Geometry: final body of the model. Coordinates: model frame, mm. A direction names the side the tool comes from. Coordinates: 2 decimals unless noted, no trailing zeros. Write each loop counter-clockwise with the first axis right and the second up, starting at its lowest first coordinate (ties: lowest second). Pieces come first, ordered by that corner, then holes. Notation, with made-up numbers: (-23, 80) -> (20, 80) arc R9 ccw to (20, 95) -> close; hole circle Ø4 at (31, 45). An arc over 180 degrees is marked (long way). One line per item, written item: value. Start each with the question number.
from build123d import *

# Parameters (mm, degrees)
SKETCH1_R             = 10.5
SKETCH1_R_2           = 7
BOSS_EXTRUDE1_DEPTH   = 90
SKETCH2_R             = 11.5
CUT_EXTRUDE1_DEPTH    = 6
SKETCH3_R             = 1.5
CUT_EXTRUDE2_DEPTH    = 40
SKETCH4_W             = 43
SKETCH4_H             = 44
CUT_EXTRUDE3_DEPTH    = 3
SKETCH5_R             = 11.5
CUT_EXTRUDE4_DEPTH    = 9
CIRPATTERN1_COUNT     = 4
SKETCH9_R             = 4
SKETCH9_R_2           = 5
CUT_EXTRUDE5_DEPTH    = 177.068168617
SKETCH10_R            = 12
CUT_EXTRUDE6_DEPTH    = 8
M4_TAPPED_HOLE1_D     = 3.3
M4_TAPPED_HOLE1_DEPTH = 19.008579979
M4_TAPPED_HOLE1_TIP   = 0.991420021


with BuildPart() as part:
    # Sketch1 → Boss-Extrude1 (new body)
    with BuildSketch(Plane.XY):
        with BuildLine():
            Line((0, 0), (64, 0))
            ThreePointArc((64, 0), (71.071067812, 2.928932188), (74, 10))
            Line((74, 10), (74, 122))
            ThreePointArc((74, 122), (71.071067812, 129.071067812), (64, 132))
            Line((64, 132), (0, 132))
            Line((0, 132), (0, 120))
            Line((0, 120), (40, 120))
            Line((40, 120), (40, 12))
            Line((40, 12), (0, 12))
            Line((0, 12), (0, 0))
        make_face()
        with Locations(Location((57, 106, 0), (0, 0, 180))):
            Circle(SKETCH1_R, mode=Mode.SUBTRACT)
        with Locations(Location((57, 66, 0), (0, 0, 180))):
            Circle(SKETCH1_R_2, mode=Mode.SUBTRACT)
        with Locations(Location((57, 26, 0), (0, 0, 180))):
            Circle(SKETCH1_R, mode=Mode.SUBTRACT)
    extrude(amount=BOSS_EXTRUDE1_DEPTH)

    # Sketch2 → Cut-Extrude1 (cut)
    with BuildSketch(Plane(origin=(0, 0, 0), x_dir=(-1, 0, 0), z_dir=(0, 0, -1))):
        with Locations((-57, 66)):
            Circle(SKETCH2_R)
    extrude(amount=-CUT_EXTRUDE1_DEPTH, mode=Mode.SUBTRACT)

    # Sketch3 → Cut-Extrude2 (cut)
    with BuildSketch(Plane(origin=(0, 0, 6), x_dir=(-1, 0, 0), z_dir=(0, 0, -1))):
        with Locations((-57, 74)):
            Circle(SKETCH3_R)
        with Locations((-49, 66)):
            Circle(SKETCH3_R)
        with Locations((-57, 58)):
            Circle(SKETCH3_R)
        with Locations((-65, 66)):
            Circle(SKETCH3_R)
    extrude(amount=-CUT_EXTRUDE2_DEPTH, mode=Mode.SUBTRACT)

    # Sketch4 → Cut-Extrude3 (cut)
    with BuildSketch(Plane(origin=(0, 132, 0), x_dir=(1, 0, 0), z_dir=(0, 1, 0))):
        with Locations((21.5, -45)):
            Rectangle(SKETCH4_W, SKETCH4_H)
    extrude(amount=-CUT_EXTRUDE3_DEPTH, mode=Mode.SUBTRACT)

    # Sketch5 → Cut-Extrude4 (cut)
    with BuildSketch(Plane(origin=(0, 129, 0), x_dir=(1, 0, 0), z_dir=(0, 1, 0))):
        with Locations(Location((21.5, -45, 0), (0, 0, 270))):
            Circle(SKETCH5_R)
    extrude(amount=-CUT_EXTRUDE4_DEPTH, mode=Mode.SUBTRACT)

    # Sketch7 → CBORE for M3 Pan Head Screw1 (revolve, cut)
    with BuildSketch(Plane(origin=(6, 120, 29.5), x_dir=(0, 0, -1), z_dir=(1, 0, 0))):
        Polygon((0, 0), (0, 21.021463052), (1.7, 20), (1.7, 3), (2.75, 3), (2.75, 0), align=None)
    cbore_for_m3_pan_head_screw1 = revolve(axis=Axis((6, 113.65, 29.5), (0, 1, 0)), mode=Mode.SUBTRACT)

    # CirPattern1: CBORE for M3 Pan Head Screw1 ×4 about axis
    cirpattern1_axis = Axis((21.5, 0, 45), (0, 1, 0))
    for i in range(1, CIRPATTERN1_COUNT):
        add(cbore_for_m3_pan_head_screw1.rotate(cirpattern1_axis, i * 360 / CIRPATTERN1_COUNT), mode=Mode.SUBTRACT)

    # Sketch9 → Cut-Extrude5 (cut, through all)
    with BuildSketch(Plane(origin=(0, 132, 0), x_dir=(1, 0, 0), z_dir=(0, 1, 0))):
        with Locations(Location((21.5, -14, 0), (0, 0, 270))):
            Circle(SKETCH9_R)
        with Locations(Location((21.5, -76, 0), (0, 0, 270))):
            Circle(SKETCH9_R)
        with Locations(Location((21.5, -45, 0), (0, 0, 270))):
            Circle(SKETCH9_R_2)
    extrude(amount=-CUT_EXTRUDE5_DEPTH, mode=Mode.SUBTRACT)

    # Sketch10 → Cut-Extrude6 (cut)
    with BuildSketch(Plane(origin=(0, 12, 0), x_dir=(1, 0, 0), z_dir=(0, 1, 0))):
        with Locations(Location((21.5, -45, 0), (0, 0, 180))):
            Circle(SKETCH10_R)
    extrude(amount=-CUT_EXTRUDE6_DEPTH, mode=Mode.SUBTRACT)

    # M4 Tapped Hole1
    with Locations(Plane.ZY):
        with Locations((14, 126), (76, 126), (76, 6), (14, 6)):
            Hole(M4_TAPPED_HOLE1_D / 2, depth=M4_TAPPED_HOLE1_DEPTH)
            with Locations((0, 0, -(M4_TAPPED_HOLE1_DEPTH + M4_TAPPED_HOLE1_TIP / 2))):  # 118° drill point
                Cone(0, M4_TAPPED_HOLE1_D / 2, M4_TAPPED_HOLE1_TIP, mode=Mode.SUBTRACT)


solid = part.part
Q1. Cut plane B-B on z = 38. Count the separate pieces of the cut face and the enclosed holes in it, and give its area (3 significant figures).
Q2. Cut plane D-D on y = 126. Output: boundary loops of the cut face in (x, z).
Q3. Draft query along Z for faces 1 (the flat face through (21, 131, 67)), 2 (the flat face through (62.3, 61, 6)), 3 (the cylindrical face through (57, 56.5, 25.7)). Return one class per face: pulls with the +Z half, pulls with the -Z half, needs draft (parallel to the pull), parting line crosses it, or undercut.
Q4. First-contact query: P1, Ø7, axis at x = 21.5, z = 76, coming from the +Y side; P2, Ø12, axis at y = 19, z = 32.5, coming from the -X side; P3, Ø1.3, axis at x = 48.5, y = 65.5, coming from the -Z side; P4, Ø7, axis at x = 26, z = 40, coming from the +Y side. Flat tips, straight axial feed; report the tip coordinate or a pass-through.
Q5. Access query for faces 4 (the flat face through (16, 12, 34)), 5 (the cylindrical face through (9.053, 5.368, 12.476)), 6 (the cylindrical face through (6.65, 125.96, 27.93)), 7 (the cylindrical face through (34.253, 121.479, 29.379)), 8 (the flat face through (43, 131, 45)). Directions: +Z, -Z, +X, -X, +Y, -Y. A direction counts if a zero-diameter tool reaches every point of the face in a straight line with its end or side. Return the directions, or none.
Q6. Cut plane A-A on y = 33. Output: boundary loops of the cut face in (x, z), and give its area (3 significant figures).
Q7. Line query: L1, parallel to Z at x = 6, y = 122.3; L2, parallel to Y at x = 57, z = 1.4; L3, parallel to Z at x = 8, y = 126. Output: solid intervals per line, ascending. Write a range as from..to.
Solution:
1. separate pieces: 2
1. enclosed holes: 3
1. area: 4,080 mm²
2. outline: (0, 0) -> (73.17, 0) -> (73.17, 90) -> (0, 90) -> (0, 77.65) -> (17.86, 77.65) arc R4 cw (long way) to (17.86, 74.35) -> (0, 74.35) -> (0, 15.65) -> (17.86, 15.65) arc R4 cw (long way) to (17.86, 12.35) -> (0, 12.35) -> close; hole circle Ø3.4 at (6, 29.5); hole circle Ø3.4 at (6, 60.5); hole circle Ø23 at (21.5, 45); hole circle Ø3.4 at (37, 29.5); hole circle Ø3.4 at (37, 60.5)
3. face 1: undercut
3. face 2: pulls with the -Z half
3. face 3: needs draft
4. P1: through
4. P2: x = 40
4. P3: z = 46
4. P4: y = 4
5. face 4: +Z, -Z, -X
5. face 5: -X
5. face 6: +Y
5. face 7: none
5. face 8: -X, +Y
6. outline: (40, 0) -> (49.17, 0) -> (49.17, 90) -> (40, 90) -> close; (64.83, 0) -> (74, 0) -> (74, 90) -> (64.83, 90) -> close
6. area: 1,650 mm²
7. L1: 0..26.75, 32.25..57.75, 63.25..90
7. L2: 0..15.5, 36.5..54.5, 77.5..95.5, 116.5..132
7. L3: 0..12.35, 15.65..74.35, 77.65..90
